Build history of the part. All positions in model axes, mm. Round coordinates to 2 decimals unless told otherwise and drop trailing zeros. Write each loop counter-clockwise with the first axis right and the second up, starting at its lowest first coordinate (ties: lowest second). Pieces come first, ordered by that corner, then holes. Notation, with made-up numbers: (70, 65) -> (110, 65) arc R17 cw to (110, 73) -> close; hole circle Ø9 at (77, -12.75). An arc over 180 degrees is marked (long way). Answer in a Markdown table with one row per item.
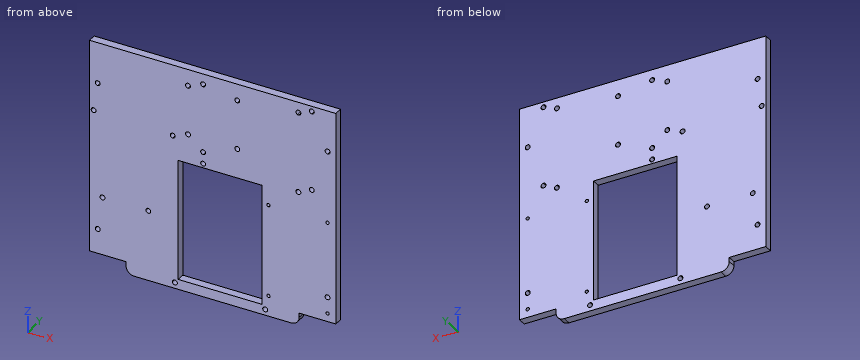
```python
from build123d import *

# Parameters (mm, degrees)
F0_W     = 105.5
F0_H     = 7.5
F1_DEPTH = 5
F3_DEPTH = 25
F4_W     = 25.1
F4_H     = 73.5
F4_W_2   = 25.9
F5_DEPTH = 25
F6_R     = 5


with BuildPart() as f1:
    # F0 (on Front) → F1 (new body)
    with BuildSketch(Plane.XZ):
        with BuildLine():
            ThreePointArc((149.692112, 105), (147.131451, 106.06066), (148.192112, 103.5))
            ThreePointArc((148.192112, 103.5), (149.252772, 103.93934), (149.692112, 105))
        make_face()
        with BuildLine():
            ThreePointArc((9.692112, 105), (7.131451, 106.06066), (8.192112, 103.5))
            ThreePointArc((8.192112, 103.5), (9.252772, 103.93934), (9.692112, 105))
        make_face()
        Polygon((3.192112, 15), (3.192112, 0), (25.442112, 0), (130.942112, 0), (153.192112, 0), (153.192112, 15), (153.192112, 130), (3.192112, 130), align=None)
        with BuildLine():
            ThreePointArc((9.692112, 15), (8.192112, 13.5), (6.692112, 15))
            ThreePointArc((6.692112, 15), (7.131451, 16.06066), (8.192112, 16.5))
            ThreePointArc((8.192112, 16.5), (9.252772, 16.06066), (9.692112, 15))
        make_face(mode=Mode.SUBTRACT)
        with BuildLine():
            ThreePointArc((148.192112, 16.5), (149.252772, 16.06066), (149.692112, 15))
            ThreePointArc((149.692112, 15), (147.131451, 13.93934), (148.192112, 16.5))
        make_face(mode=Mode.SUBTRACT)
        with BuildLine():
            ThreePointArc((9.692112, 105), (9.252772, 103.93934), (8.192112, 103.5))
            ThreePointArc((8.192112, 103.5), (7.131451, 106.06066), (9.692112, 105))
        make_face(mode=Mode.SUBTRACT)
        with BuildLine():
            ThreePointArc((149.692112, 105), (149.252772, 103.93934), (148.192112, 103.5))
            ThreePointArc((148.192112, 103.5), (147.131451, 106.06066), (149.692112, 105))
        make_face(mode=Mode.SUBTRACT)
        with Locations((78.192112, -3.75)):
            Rectangle(F0_W, F0_H)
    extrude(amount=F1_DEPTH)

    # F2 (on face) → F3 (cut)
    with BuildSketch(Plane.XZ.offset(5)):
        with BuildLine():
            ThreePointArc((7.192112, 87.6), (5.692112, 89.1), (4.192112, 87.6))
            Line((4.192112, 87.6), (5.692112, 87.6))
            Line((5.692112, 87.6), (5.692112, 86.3))
            Line((5.692112, 86.3), (6.440443, 86.3))
            ThreePointArc((6.440443, 86.3), (6.990668, 86.849166), (7.192112, 87.6))
        make_face()
        with BuildLine():
            ThreePointArc((12.60054, 35.331822), (12.600533, 35.336368), (12.600512, 35.340914))
            ThreePointArc((12.600512, 35.340914), (9.600547, 35.327276), (12.60054, 35.331822))
        make_face()
        with BuildLine():
            ThreePointArc((40.500027, 35.500933), (40.50002, 35.505479), (40.5, 35.510025))
            Line((40.5, 35.510025), (39.000027, 35.500933))
            Line((39.000027, 35.500933), (37.500055, 35.491841))
            ThreePointArc((37.500055, 35.491841), (39.004573, 34.00094), (40.500027, 35.500933))
        make_face()
        with BuildLine():
            Line((39.000027, 35.500933), (40.5, 35.510025))
            ThreePointArc((40.5, 35.510025), (38.990935, 37.000906), (37.500055, 35.491841))
            Line((37.500055, 35.491841), (39.000027, 35.500933))
        make_face()
        with BuildLine():
            ThreePointArc((55.391832, 86.392132), (53.887286, 87.892125), (52.39186, 86.38304))
            Line((52.39186, 86.38304), (53.891832, 86.392132))
            Line((53.891832, 86.392132), (53.900924, 84.89216))
            ThreePointArc((53.900924, 84.89216), (54.955702, 85.334691), (55.391832, 86.392132))
        make_face()
        with BuildLine():
            Line((53.891832, 86.392132), (52.39186, 86.38304))
            ThreePointArc((52.39186, 86.38304), (52.837621, 85.325063), (53.900924, 84.89216))
            Line((53.900924, 84.89216), (53.891832, 86.392132))
        make_face()
        with BuildLine():
            Line((5.692112, 87.6), (4.192112, 87.6))
            ThreePointArc((4.192112, 87.6), (4.941278, 86.301444), (6.440443, 86.3))
            Line((6.440443, 86.3), (5.692112, 86.3))
            Line((5.692112, 86.3), (5.692112, 87.6))
        make_face()
        with BuildLine():
            ThreePointArc((147.192112, 5), (148.192112, 4), (149.192112, 5))
            Line((149.192112, 5), (148.192112, 5))
            Line((148.192112, 5), (147.192112, 5))
        make_face()
        with BuildLine():
            Line((148.192112, 5), (149.192112, 5))
            ThreePointArc((149.192112, 5), (148.192112, 6), (147.192112, 5))
            Line((147.192112, 5), (148.192112, 5))
        make_face()
        with BuildLine():
            ThreePointArc((149.192112, 61), (148.192112, 62), (147.192112, 61))
            ThreePointArc((147.192112, 61), (148.192112, 60), (149.192112, 61))
        make_face()
        with BuildLine():
            ThreePointArc((113.192112, 61), (111.485005, 61.707107), (112.192112, 60))
            Line((112.192112, 60), (112.192112, 61))
            Line((112.192112, 61), (113.192112, 61))
        make_face()
        with BuildLine():
            Line((112.192112, 61), (112.192112, 60))
            ThreePointArc((112.192112, 60), (112.899218, 60.292893), (113.192112, 61))
            Line((113.192112, 61), (112.192112, 61))
        make_face()
        with BuildLine():
            ThreePointArc((112.192112, 6), (111.485005, 4.292893), (113.192112, 5))
            Line((113.192112, 5), (112.192112, 5))
            Line((112.192112, 5), (112.192112, 6))
        make_face()
        with BuildLine():
            Line((112.192112, 5), (113.192112, 5))
            ThreePointArc((113.192112, 5), (112.899218, 5.707107), (112.192112, 6))
            Line((112.192112, 6), (112.192112, 5))
        make_face()
        with BuildLine():
            ThreePointArc((140.082112, 78.43), (139.642772, 79.49066), (138.582112, 79.93))
            ThreePointArc((138.582112, 79.93), (137.521451, 77.36934), (140.082112, 78.43))
        make_face()
        with BuildLine():
            ThreePointArc((140.082112, 126.82), (139.642772, 127.88066), (138.582112, 128.32))
            Line((138.582112, 128.32), (138.582112, 126.82))
            Line((138.582112, 126.82), (138.582112, 125.32))
            ThreePointArc((138.582112, 125.32), (139.642772, 125.75934), (140.082112, 126.82))
        make_face()
        with BuildLine():
            Line((138.582112, 126.82), (138.582112, 128.32))
            ThreePointArc((138.582112, 128.32), (137.082112, 126.82), (138.582112, 125.32))
            Line((138.582112, 125.32), (138.582112, 126.82))
        make_face()
        with BuildLine():
            ThreePointArc((64.692112, 90), (64.252772, 91.06066), (63.192112, 91.5))
            ThreePointArc((63.192112, 91.5), (62.131451, 88.93934), (64.692112, 90))
        make_face()
        with BuildLine():
            ThreePointArc((64.692112, 120), (62.131451, 121.06066), (63.192112, 118.5))
            ThreePointArc((63.192112, 118.5), (64.252772, 118.93934), (64.692112, 120))
        make_face()
        with BuildLine():
            ThreePointArc((72.422112, 125.15), (70.922112, 123.65), (72.422112, 122.15))
            Line((72.422112, 122.15), (72.422112, 123.65))
            Line((72.422112, 123.65), (72.422112, 125.15))
        make_face()
        with BuildLine():
            Line((72.422112, 123.65), (72.422112, 122.15))
            ThreePointArc((72.422112, 122.15), (73.482772, 122.58934), (73.922112, 123.65))
            ThreePointArc((73.922112, 123.65), (73.482772, 124.71066), (72.422112, 125.15))
            Line((72.422112, 125.15), (72.422112, 123.65))
        make_face()
        with BuildLine():
            ThreePointArc((72.422112, 83.24), (70.922112, 81.74), (72.422112, 80.24))
            Line((72.422112, 80.24), (72.422112, 81.74))
            Line((72.422112, 81.74), (72.422112, 83.24))
        make_face()
        with BuildLine():
            Line((72.422112, 81.74), (72.422112, 80.24))
            ThreePointArc((72.422112, 80.24), (73.482772, 80.67934), (73.922112, 81.74))
            ThreePointArc((73.922112, 81.74), (73.482772, 82.80066), (72.422112, 83.24))
            Line((72.422112, 83.24), (72.422112, 81.74))
        make_face()
        with BuildLine():
            ThreePointArc((72.422112, 76.15), (71.361451, 73.58934), (73.922112, 74.65))
            Line((73.922112, 74.65), (72.422112, 74.65))
            Line((72.422112, 74.65), (72.422112, 76.15))
        make_face()
        with BuildLine():
            Line((72.422112, 74.65), (73.922112, 74.65))
            ThreePointArc((73.922112, 74.65), (73.482772, 75.71066), (72.422112, 76.15))
            Line((72.422112, 76.15), (72.422112, 74.65))
        make_face()
        with BuildLine():
            ThreePointArc((131.922112, 74.65), (131.482772, 75.71066), (130.422112, 76.15))
            Line((130.422112, 76.15), (130.422112, 74.65))
            Line((130.422112, 74.65), (128.922112, 74.65))
            ThreePointArc((128.922112, 74.65), (130.422112, 73.15), (131.922112, 74.65))
        make_face()
        with BuildLine():
            Line((130.422112, 74.65), (130.422112, 76.15))
            ThreePointArc((130.422112, 76.15), (129.361451, 75.71066), (128.922112, 74.65))
            Line((128.922112, 74.65), (130.422112, 74.65))
        make_face()
        with BuildLine():
            ThreePointArc((131.922112, 123.65), (131.182046, 124.943252), (129.692112, 124.960382))
            Line((129.692112, 124.960382), (129.692112, 122.339618))
            ThreePointArc((129.692112, 122.339618), (130.044999, 122.198178), (130.422112, 122.15))
            ThreePointArc((130.422112, 122.15), (131.482772, 122.58934), (131.922112, 123.65))
        make_face()
        with BuildLine():
            Line((129.692112, 122.339618), (129.692112, 124.960382))
            ThreePointArc((129.692112, 124.960382), (128.922112, 123.65), (129.692112, 122.339618))
        make_face()
        with BuildLine():
            ThreePointArc((93.192112, 91.5), (92.131451, 88.93934), (94.692112, 90))
            ThreePointArc((94.692112, 90), (94.252772, 91.06066), (93.192112, 91.5))
        make_face()
        with BuildLine():
            ThreePointArc((93.192112, 121.5), (91.692112, 120), (93.192112, 118.5))
            Line((93.192112, 118.5), (93.192112, 120))
            Line((93.192112, 120), (93.192112, 121.5))
        make_face()
        with BuildLine():
            Line((93.192112, 120), (93.192112, 118.5))
            ThreePointArc((93.192112, 118.5), (94.252772, 118.93934), (94.692112, 120))
            ThreePointArc((94.692112, 120), (94.252772, 121.06066), (93.192112, 121.5))
            Line((93.192112, 121.5), (93.192112, 120))
        make_face()
    extrude(amount=-F3_DEPTH, mode=Mode.SUBTRACT)

    # F4 (on face) → F5 (cut)
    with BuildSketch(Plane(origin=(0, 0, 0), x_dir=(-1, 0, 0), z_dir=(0, 1, 0))):
        with Locations((-95.642112, 35.35)):
            Rectangle(F4_W, F4_H)
        with Locations((-70.142112, 35.35)):
            Rectangle(F4_W_2, F4_H)
        with BuildLine():
            ThreePointArc((-108.692112, -3.9), (-109.131451, -2.83934), (-110.192112, -2.4))
            ThreePointArc((-110.192112, -2.4), (-111.252772, -4.96066), (-108.692112, -3.9))
        make_face()
        with BuildLine():
            ThreePointArc((-53.692112, -3.9), (-54.131451, -2.83934), (-55.192112, -2.4))
            ThreePointArc((-55.192112, -2.4), (-56.252772, -4.96066), (-53.692112, -3.9))
        make_face()
    extrude(amount=-F5_DEPTH, mode=Mode.SUBTRACT)

    # F6
    f6_edges = [f1.edges().sort_by_distance(p)[0] for p in [
        (130.942112, -2.5, -7.5),
        (25.442112, -2.5, -7.5),
    ]]
    fillet(f6_edges, radius=F6_R)


solid = f1.part
```
Q1. Drop flat-ended pins along their axis: P1, Ø1.5, axis at x = 126.5, z = 13, coming from the +Y side; P2, Ø0.8, axis at y = -2, z = -1, coming from the +X side. Give the stop position or say it passes through.
A:
| item | result |
|---|---|
| P1 | y = 0 |
| P2 | x = 130.94 |
Q2. Wall check: line 1 (X direction, y = -3.65, z = 120); line 2 (X direction, y = -3.55, z = 105); line 3 (Z direction, x = 96, y = -2.2). Give the ranges that are in metal, low to high. Write a range as [from, to].
A:
| item | result |
|---|---|
| line 1 | [3.19, 61.69], [64.69, 91.69], [94.69, 153.19] |
| line 2 | [3.19, 6.69], [9.69, 146.69], [149.69, 153.19] |
| line 3 | [-7.5, -1.4], [72.1, 130] |
Q3. Saw through at C-C on y = -2.9. State how many separate pieces and enclosed holes the cut face has, plus the area to 3 significant figures.
A:
| item | result |
|---|---|
| separate pieces | 1 |
| enclosed holes | 26 |
| area | 16,400 mm² |
Q4. Saw through at A-A on z = 45. Write the cut outline in (x, y).
A:
| item | result |
|---|---|
| outline | (3.19, -5) -> (57.19, -5) -> (57.19, 0) -> (3.19, 0) -> close; (108.19, -5) -> (153.19, -5) -> (153.19, 0) -> (108.19, 0) -> close |
Q5. Saw through at D-D on x = 18.5. Write the cut outline in (y, z), plus the area to 3 significant figures.
A:
| item | result |
|---|---|
| outline | (-5, 0) -> (0, 0) -> (0, 130) -> (-5, 130) -> close |
| area | 650 mm² |
Q6. Saw through at B-B on x = 88.5. Write the cut outline in (y, z).
A:
| item | result |
|---|---|
| outline | (-5, -7.5) -> (0, -7.5) -> (0, -1.4) -> (-5, -1.4) -> close; (-5, 72.1) -> (0, 72.1) -> (0, 130) -> (-5, 130) -> close |
